The drawing under review shows one solid part. Ordinate dimensions are in mm from its lowest x, y, z. Coordinates: 2 decimals unless noted, no trailing zeros. Loops run counter-clockwise (first coordinate to the right, second up) from the corner with the lowest first, then second, coordinate; pieces in that order, holes last. Notation, with made-up numbers: M 36,-27.75 L 69,-27.75 A28 cw 69,2.25 Z; hole C -31.5,32 d8. An arc over 180 degrees is marked long. Answer as a JSON object with one key per item and string values. Group by question number.
1. Consider section B-B (x = 19). State the section outline as (y, z) points.
2. To check wall thickness, follow probe 1 along X at (y, z) = (8.5, 1); probe 2 along Y at (x, z) = (31, 1.5); probe 3 along X at (y, z) = (4.25, 0.7). State the ranges of each line that lie inside material, in increasing order.
3. Consider section A-A (y = 6.5). State the section outline as (x, z) points, then the cut area to 3 significant figures.
4. Draft analysis for pull direction X (two halves, no side actions). For the marked faces 1, 2, 3 and 4, state which applies: +X half, -X half, draft (parallel to the pull), parting line (faces both ways), or undercut.
5. Consider section D-D (x = 31). State the section outline as (y, z) points.
6. Consider section C-C (z = 4.9). State the section outline as (x, y) points.
7. Insertion check: pin 1 (3 mm diameter, centred on x = 7, y = 6.5, fed in from -Z). The pin has a flat end and moves straight along its axis. Give the tip position at first contact, or say it passes through.
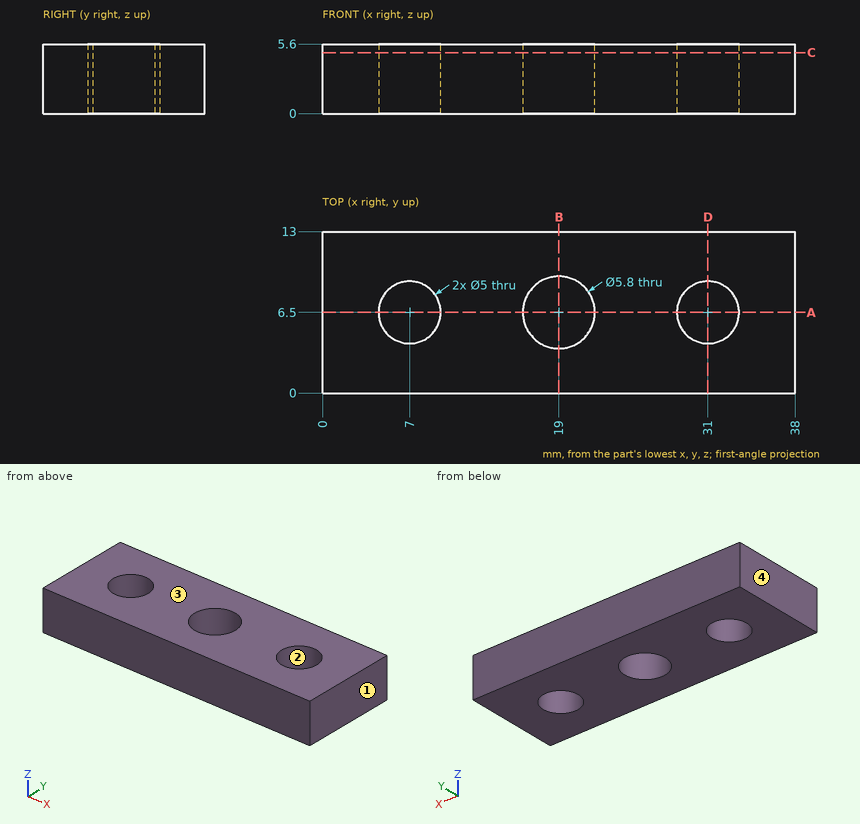
Findings below:
{
 "1": {"outline": "M 0,0 L 3.6,0 L 3.6,5.6 L 0,5.6 Z; M 9.4,0 L 13,0 L 13,5.6 L 9.4,5.6 Z"},
 "2": {"probe 1": "x = 0 to 5.5, 8.5 to 16.9, 21.1 to 29.5, 32.5 to 38", "probe 2": "y = 0 to 4, 9 to 13", "probe 3": "x = 0 to 5.91, 8.09 to 17.17, 20.83 to 29.91, 32.09 to 38"},
 "3": {"outline": "M 0,0 L 4.5,0 L 4.5,5.6 L 0,5.6 Z; M 9.5,0 L 16.1,0 L 16.1,5.6 L 9.5,5.6 Z; M 21.9,0 L 28.5,0 L 28.5,5.6 L 21.9,5.6 Z; M 33.5,0 L 38,0 L 38,5.6 L 33.5,5.6 Z", "area": "124 mm^2"},
 "4": {"face 1": "+X half", "face 2": "undercut", "face 3": "draft", "face 4": "-X half"},
 "5": {"outline": "M 0,0 L 4,0 L 4,5.6 L 0,5.6 Z; M 9,0 L 13,0 L 13,5.6 L 9,5.6 Z"},
 "6": {"outline": "M 0,0 L 38,0 L 38,13 L 0,13 Z; hole C 7,6.5 d5; hole C 19,6.5 d5.8; hole C 31,6.5 d5"},
 "7": {"pin 1": "passes through"}
}
